For this review, take the finished solid that the model builds, in its own axes (mm). Face numbers are marked on the shaded views. A direction names the side the tool comes from. Round coordinates to 2 decimals unless told otherwise and drop trailing zeros. Order: outer loops, then holes, each group sorted by start corner. A loop starts at its lowest first (then second) coordinate and runs counter-clockwise, first axis right, second up.
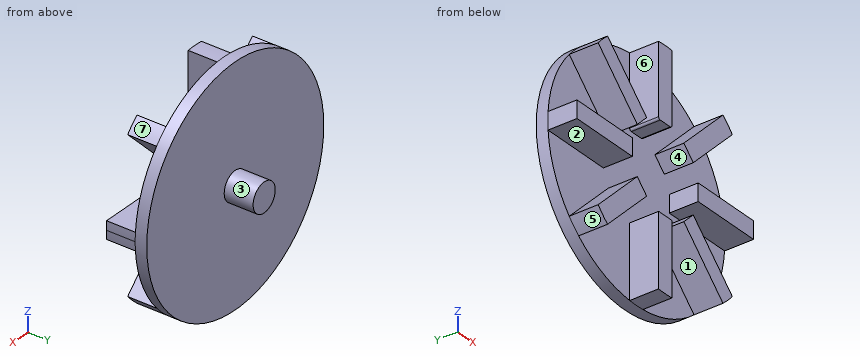
from build123d import *

# Parameters (mm, degrees)
F0_R     = 20
F1_DEPTH = 2
F3_DEPTH = 5
F4_R     = 2.5
F5_DEPTH = 5


with BuildPart() as f1:
    # F0 (on Front) → F1 (new body)
    with BuildSketch(Plane.XZ):
        Circle(F0_R)
    extrude(amount=F1_DEPTH)

    # F2 (on face) → F3 (join)
    with BuildSketch(Plane.XZ.offset(2)):
        with BuildLine():
            Line((-4.20281, 6.32413), (-13.041645, 15.162965))
            ThreePointArc((-13.041645, 15.162965), (-14.142136, 14.142136), (-15.162965, 13.041645))
            Line((-15.162965, 13.041645), (-6.32413, 4.20281))
            Line((-6.32413, 4.20281), (-5.26347, 5.26347))
            Line((-5.26347, 5.26347), (-4.20281, 6.32413))
        make_face()
        with BuildLine():
            Line((-7.443671, 1.5), (-19.943671, 1.5))
            ThreePointArc((-19.943671, 1.5), (-20, 0), (-19.943671, -1.5))
            Line((-19.943671, -1.5), (-7.443671, -1.5))
            Line((-7.443671, -1.5), (-7.443671, 0))
            Line((-7.443671, 0), (-7.443671, 1.5))
        make_face()
        with BuildLine():
            Line((-6.32413, -4.20281), (-15.162965, -13.041645))
            ThreePointArc((-15.162965, -13.041645), (-14.142136, -14.142136), (-13.041645, -15.162965))
            Line((-13.041645, -15.162965), (-4.20281, -6.32413))
            Line((-4.20281, -6.32413), (-5.26347, -5.26347))
            Line((-5.26347, -5.26347), (-6.32413, -4.20281))
        make_face()
        with BuildLine():
            Line((-1.5, -7.443671), (-1.5, -19.943671))
            ThreePointArc((-1.5, -19.943671), (0, -20), (1.5, -19.943671))
            Line((1.5, -19.943671), (1.5, -7.443671))
            Line((1.5, -7.443671), (0, -7.443671))
            Line((0, -7.443671), (-1.5, -7.443671))
        make_face()
        with BuildLine():
            ThreePointArc((-1.5, 7.805948), (-1.393892, 7.549779), (-1.137723, 7.443671))
            Line((-1.137723, 7.443671), (0, 7.443671))
            Line((0, 7.443671), (1.137723, 7.443671))
            ThreePointArc((1.137723, 7.443671), (1.393892, 7.549779), (1.5, 7.805948))
            Line((1.5, 7.805948), (1.5, 19.943671))
            ThreePointArc((1.5, 19.943671), (0, 20), (-1.5, 19.943671))
            Line((-1.5, 19.943671), (-1.5, 7.805948))
        make_face()
        with BuildLine():
            ThreePointArc((15.162965, 13.041645), (14.142136, 14.142136), (13.041645, 15.162965))
            Line((13.041645, 15.162965), (4.20281, 6.32413))
            Line((4.20281, 6.32413), (5.26347, 5.26347))
            Line((5.26347, 5.26347), (6.32413, 4.20281))
            Line((6.32413, 4.20281), (15.162965, 13.041645))
        make_face()
        with BuildLine():
            ThreePointArc((20, 0), (19.985913, 0.750529), (19.943671, 1.5))
            Line((19.943671, 1.5), (7.443671, 1.5))
            Line((7.443671, 1.5), (7.443671, 0))
            Line((7.443671, 0), (7.443671, -1.5))
            Line((7.443671, -1.5), (19.943671, -1.5))
            ThreePointArc((19.943671, -1.5), (19.985913, -0.750529), (20, 0))
        make_face()
        with BuildLine():
            ThreePointArc((13.041645, -15.162965), (14.142136, -14.142136), (15.162965, -13.041645))
            Line((15.162965, -13.041645), (6.32413, -4.20281))
            Line((6.32413, -4.20281), (5.26347, -5.26347))
            Line((5.26347, -5.26347), (4.20281, -6.32413))
            Line((4.20281, -6.32413), (13.041645, -15.162965))
        make_face()
    extrude(amount=F3_DEPTH)

    # F4 (on face) → F5 (join)
    with BuildSketch(Plane.XZ):
        Circle(F4_R)
    extrude(amount=-F5_DEPTH)


solid = f1.part
(1) Add section D-D on x = 9. Give the boundary of the cut face in (y, z).
(2) Wall thickness on L1, parallel to X at y = -6, z = 9.5; L2, parallel to X at y = -3, z = 10; L3, parallel to Z at x = 13, y = -4.25: over which ranges is each line inside the solid? List them lowest first.
(3) Draft analysis for pull direction X (two halves, no side actions). For the marked faces 5, 6 and 7, state which applies: pulls with the +X half, pulls with the -X half, needs draft (parallel to the pull), parting line crosses it, or undercut.
(4) Tool access review of the marked faces 1, 2, 3 and 4: name each direction out of +Z, -Z, +X, -X, +Y, -Y from which nothing blocks a thin tool from reaching the whole face with its end or side.
(5) Add section C-C on z = -14.5. Give the boundary of the cut face in (x, y).
(6) Clearance check with flat-ended pins moving along their axes: P1, Ø5.5, axis at y = -4, z = -12, coming from the -X side; P2, Ø2.5, axis at x = -13.5, y = -5.5, coming from the +Z side; P3, Ø1.5, axis at x = -4, z = 12.5, coming from the -Y side. State where each tip first meets the part, or that it passes through.
(7) Add section B-B on y = -2.5. Count the separate pieces of the cut face and the enclosed holes in it, plus the area to 3 significant figures.
(8) Add section A-A on x = 0. Give the boundary of the cut face in (y, z).
Here are the results:
1. outline: (-7, -11.12) - (-2, -11.12) - (-2, -17.86) - (0, -17.86) - (0, 17.86) - (-2, 17.86) - (-2, 11.12) - (-7, 11.12) - (-7, 6.88) - (-2, 6.88) - (-2, 1.5) - (-7, 1.5) - (-7, -1.5) - (-2, -1.5) - (-2, -6.88) - (-7, -6.88) - close
2. L1: x = -11.62 to -7.38, -1.5 to 1.5, 7.38 to 11.62
2. L2: x = -12.12 to -7.88, -1.5 to 1.5, 7.88 to 12.12
2. L3: z = -15.12 to -10.88, -1.5 to 1.5, 10.88 to 15.12
3. face 5: pulls with the -X half
3. face 6: undercut
3. face 7: pulls with the +X half
4. face 1: -Z, -Y
4. face 2: +X, -X, -Y
4. face 3: +Y
4. face 4: -Y
5. outline: (-13.77, -7) - (-12.38, -7) - (-12.38, -2) - (-1.5, -2) - (-1.5, -7) - (1.5, -7) - (1.5, -2) - (12.38, -2) - (12.38, -7) - (13.77, -7) - (13.77, 0) - (-13.77, 0) - close
6. P1: stops at x = -17.26
6. P2: stops at z = 15.16
6. P3: stops at y = -2
7. separate pieces: 8
7. enclosed holes: 0
7. area: 301 mm2
8. outline: (-7, -20) - (0, -20) - (0, -2.5) - (5, -2.5) - (5, 2.5) - (0, 2.5) - (0, 20) - (-7, 20) - (-7, 7.44) - (-2, 7.44) - (-2, -7.44) - (-7, -7.44) - close
